from build123d import *

# Parameters (mm, degrees)
F1_DEPTH      = 24
F3_START      = 24
F2_W          = 89
F2_H          = 60
F3_DEPTH      = 5
F4_DEPTH      = 5
F5_R          = 2.75
F6_DEPTH      = 29.001
F6_DEPTH_BACK = 5.001
F7_W          = 77
F7_H          = 5.5
F8_DEPTH      = 5
F8_DEPTH_BACK = 2
F10_START     = 22
F10_DEPTH     = 7


with BuildPart() as f1:
    # F0 (on Front) → F1 (new body)
    with BuildSketch(Plane.XZ):
        Polygon((12, 60), (-77, 60), (-77, 0), (-65, 0), (-65, 55), (0, 55), (0, 0), (12, 0), align=None)
    extrude(amount=F1_DEPTH)

    # F2 (on Front) → F3 (join)
    with BuildSketch(Plane.XZ.offset(F3_START)):
        with Locations((-32.5, 30)):
            Rectangle(F2_W, F2_H)
    extrude(amount=F3_DEPTH)

    # F2 (on Front) → F4 (join)
    with BuildSketch(Plane.XZ):
        with Locations((-32.5, 30)):
            Rectangle(F2_W, F2_H)
    extrude(amount=-F4_DEPTH)

    # F5 (on Front) → F6 (cut, two sides)
    with BuildSketch(Plane.XZ) as f6_sk:
        with Locations((-71, 25)):
            Circle(F5_R)
        with Locations((-71, 10)):
            Circle(F5_R)
        with Locations((6, 10)):
            Circle(F5_R)
        with Locations((6, 25)):
            Circle(F5_R)
        with Locations((6, 40)):
            Circle(F5_R)
        with Locations((-71, 40)):
            Circle(F5_R)
    extrude(amount=F6_DEPTH, mode=Mode.SUBTRACT)
    extrude(f6_sk.sketch, amount=-F6_DEPTH_BACK, mode=Mode.SUBTRACT)

    # F7 (on Front) → F8 (cut, two sides)
    with BuildSketch(Plane.XZ) as f8_sk:
        with Locations((-32.5, 40)):
            Rectangle(F7_W, F7_H)
        with Locations((-32.5, 25)):
            Rectangle(F7_W, F7_H)
        with Locations((-32.5, 10)):
            Rectangle(F7_W, F7_H)
    extrude(amount=-F8_DEPTH, mode=Mode.SUBTRACT)
    extrude(f8_sk.sketch, amount=F8_DEPTH_BACK, mode=Mode.SUBTRACT)

    # F9 (on Front) → F10 (cut)
    with BuildSketch(Plane.XZ.offset(F10_START)):
        Polygon((-70.4741701855, 27.6992597145), (-71.5258298145, 22.3007402855), (5.4741701855, 7.3007402855), (6.5258298145, 12.6992597145), align=None)
        Polygon((-70.4741701855, 42.6992597145), (-71.5258298145, 37.3007402855), (5.4741701855, 22.3007402855), (6.5258298145, 27.6992597145), align=None)
    extrude(amount=F10_DEPTH, mode=Mode.SUBTRACT)


solid = f1.part
Design review of the part built by this model. Coordinates are the model's own, in mm. A direction names the side the tool comes from. Round coordinates to 2 decimals unless told otherwise and drop trailing zeros. Write each loop counter-clockwise with the first axis right and the second up, starting at its lowest first coordinate (ties: lowest second). Pieces come first, ordered by that corner, then holes. Notation, with made-up numbers: (80.5, -11.5) -> (93.5, -11.5) arc R15 cw to (93.5, 7.5) -> close; hole circle Ø6 at (63, 13). An arc over 180 degrees is marked (long way). One line per item, written item: value. Start each with the question number.
Q1. Insertion check: P1, Ø3.5, axis at x = 6, z = 10, coming from the +Y side; P2, Ø3.5, axis at x = 4.5, z = 25.5, coming from the -Y side; P3, Ø3, axis at x = 3.5, z = 11, coming from the +Y side. Each pin has a flat end and moves straight along its axis. Give the tip position at first contact, or say it passes through.
Q2. Tool access review of faces 4 (the face through (-33, -24, 45)), 5 (the face through (-67, -2, 40)), 6 (the face through (-33.565, -26.229, 14.906)): name each direction out of +Z, -Z, +X, -X, +Y, -Y from which nothing blocks a thin tool from reaching the whole face with its end or side.
Q3. Add section D-D (z = 10). Give the boundary of the cut face in (x, y).
Q4. The part is to be moulded in two halves that separate along Z. For faces 1 (the face through (-33, 2, 12.75)), 2 (the face through (12, -12, 30)), 3 (the face through (-33, -12, 60)), say which applies: pulls with the +Z half, pulls with the -Z half, needs draft (parallel to the pull), parting line crosses it, or undercut.
Q5. To check wall thickness, follow probe 1 along Z at (x, y) = (6, -11.5); probe 2 along X at (y, z) = (-19.5, 40); probe 3 along X at (y, z) = (-14.5, 22). State the ranges of each line that lie inside material, in increasing order.
Q6. Add section C-C (x = -3). Give the boundary of the cut face in (y, z), then the cut area to 3 significant figures.
Q7. Add section B-B (y = -19). Give the boundary of the cut face in (x, z).
Q8. Add section A-A (z = 25). Give the boundary of the cut face in (x, y).
Response:
1. P1: passes through
1. P2: stops at y = -22
1. P3: stops at y = -2
2. face 4: -Z
2. face 5: +Y
2. face 6: -Y
3. outline: (-77, -29) -> (-73.75, -29) -> (-73.75, 5) -> (-77, 5) -> close; (-68.25, -29) -> (-8.38, -29) -> (-8.38, -24) -> (-65, -24) -> (-65, -2) -> (-68.25, -2) -> close; (0, -22) -> (3.25, -22) -> (3.25, -2) -> (0, -2) -> close; (8.75, -29) -> (12, -29) -> (12, 5) -> (8.75, 5) -> close
4. face 1: undercut
4. face 2: needs draft
4. face 3: pulls with the +Z half
5. probe 1: z = 0 to 7.25, 12.75 to 22.25, 27.75 to 37.25, 42.75 to 60
5. probe 2: x = -77 to -73.75, -68.25 to -65, 0 to 3.25, 8.75 to 12
5. probe 3: x = -77 to -65, 0 to 12
6. outline: (-29, 0) -> (-24, 0) -> (-24, 8.95) -> (-29, 8.95) -> close; (-29, 14.55) -> (-24, 14.55) -> (-24, 23.95) -> (-29, 23.95) -> close; (-29, 29.55) -> (-24, 29.55) -> (-24, 55) -> (0, 55) -> (0, 42.75) -> (5, 42.75) -> (5, 60) -> (-29, 60) -> close; (0, 0) -> (5, 0) -> (5, 7.25) -> (0, 7.25) -> close; (0, 12.75) -> (5, 12.75) -> (5, 22.25) -> (0, 22.25) -> close; (0, 27.75) -> (5, 27.75) -> (5, 37.25) -> (0, 37.25) -> close
6. area: 581 mm^2
7. outline: (-77, 0) -> (-65, 0) -> (-65, 55) -> (0, 55) -> (0, 0) -> (12, 0) -> (12, 60) -> (-77, 60) -> close; hole circle Ø5.5 at (-71, 10); hole circle Ø5.5 at (-71, 25); hole circle Ø5.5 at (-71, 40); hole circle Ø5.5 at (6, 10); hole circle Ø5.5 at (6, 25); hole circle Ø5.5 at (6, 40)
8. outline: (-77, -29) -> (-73.75, -29) -> (-73.75, 5) -> (-77, 5) -> close; (-68.25, -22) -> (-65, -22) -> (-65, -2) -> (-68.25, -2) -> close; (-56.62, -29) -> (-8.38, -29) -> (-8.38, -24) -> (-56.62, -24) -> close; (0, -22) -> (3.25, -22) -> (3.25, -2) -> (0, -2) -> close; (8.75, -29) -> (12, -29) -> (12, 5) -> (8.75, 5) -> close
